Design review of the part shown in the three views and the two pictorial views. Dimensions are in mm from the part's minimum x, y and z. A direction names the side the tool comes from. Give positions to 0.01 mm unless a question says otherwise; leave off trailing zeros. Order: outer loops, then holes, each group sorted by start corner. A loop starts at its lowest first (then second) coordinate and runs counter-clockwise, first axis right, second up. Notation, with made-up numbers: (60, 76.25) -> (101, 76.25) arc R25 ccw to (101, 90.25) -> close; hole circle Ø10 at (69, 25). An arc over 180 degrees is marked (long way). Use one line per item in the form item = value.
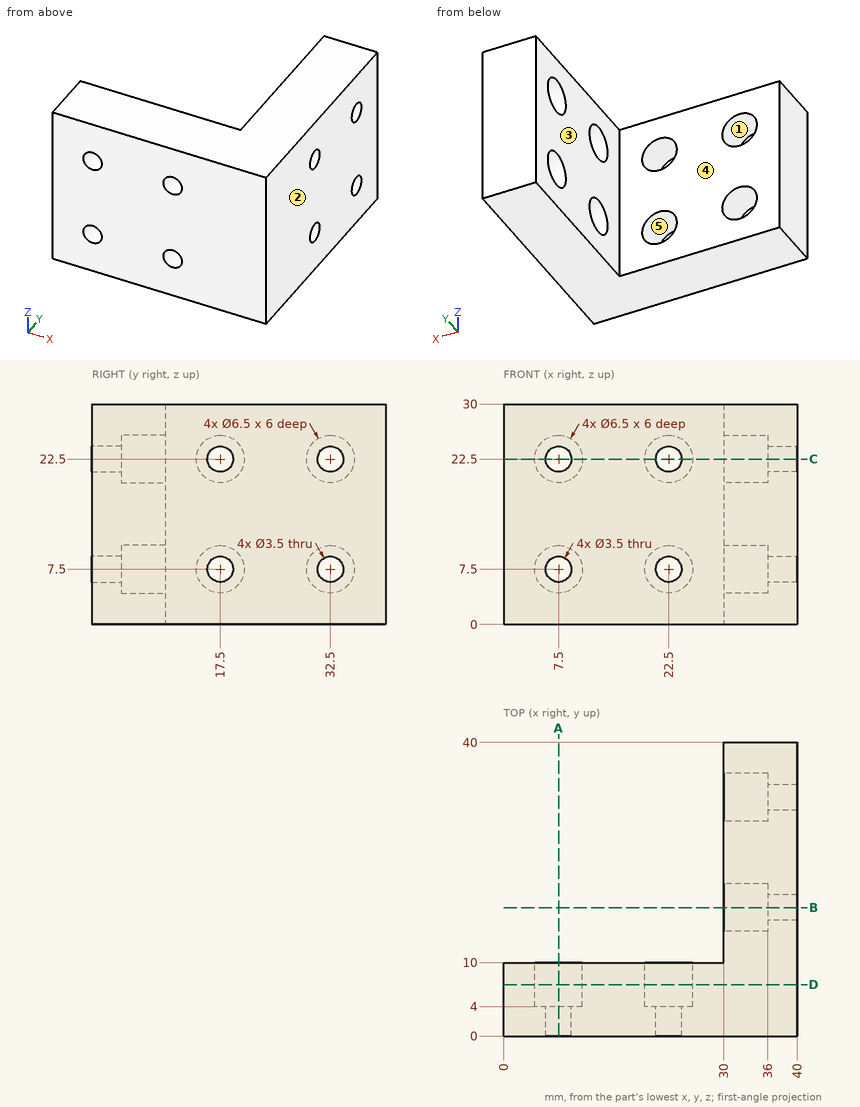
1. Add section C-C on z = 22.5. Count the separate pieces of the cut face and the enclosed holes in it, then the cut area to 3 significant figures.
Values:
separate_pieces = 5
enclosed_holes = 0
area = 488 mm^2
2. Tool access review of the marked faces 1 and 2: name each direction out of +Z, -Z, +X, -X, +Y, -Y from which nothing blocks a thin tool from reaching the whole face with its end or side.
Values:
face_1 = +Y
face_2 = +Z, -Z, +X, +Y, -Y
3. Add section D-D on y = 7. Give the boundary of the cut face in (x, z).
Values:
outline = (0, 0) -> (40, 0) -> (40, 30) -> (0, 30) -> close; hole circle Ø6.5 at (7.5, 7.5); hole circle Ø6.5 at (7.5, 22.5); hole circle Ø6.5 at (22.5, 7.5); hole circle Ø6.5 at (22.5, 22.5)
4. Add section A-A on x = 7.5. Give the boundary of the cut face in (y, z).
Values:
outline = (0, 0) -> (10, 0) -> (10, 4.25) -> (4, 4.25) -> (4, 5.75) -> (0, 5.75) -> close; (0, 9.25) -> (4, 9.25) -> (4, 10.75) -> (10, 10.75) -> (10, 19.25) -> (4, 19.25) -> (4, 20.75) -> (0, 20.75) -> close; (0, 24.25) -> (4, 24.25) -> (4, 25.75) -> (10, 25.75) -> (10, 30) -> (0, 30) -> close
5. For L1, parallel to Y at x = 37.35, z = 22.5; L2, parallel to X at y = 1, z = 22.5; L3, parallel to X at y = 6.05, z = 7.5, list the stretches that pass through material, from the lowest coordinate up.
Values:
L1 = 0 to 15.75, 19.25 to 30.75, 34.25 to 40
L2 = 0 to 5.75, 9.25 to 20.75, 24.25 to 40
L3 = 0 to 4.25, 10.75 to 19.25, 25.75 to 40
6. The part is to be moulded in two halves that separate along X. For the marked faces 3, 4 and 5, say which applies: +X half, -X half, draft (parallel to the pull), parting line (faces both ways), or undercut.
Values:
face_3 = -X half
face_4 = draft
face_5 = undercut
7. Add section B-B on y = 17.5. Give the boundary of the cut face in (x, z).
Values:
outline = (30, 0) -> (40, 0) -> (40, 5.75) -> (36, 5.75) -> (36, 4.25) -> (30, 4.25) -> close; (30, 10.75) -> (36, 10.75) -> (36, 9.25) -> (40, 9.25) -> (40, 20.75) -> (36, 20.75) -> (36, 19.25) -> (30, 19.25) -> close; (30, 25.75) -> (36, 25.75) -> (36, 24.25) -> (40, 24.25) -> (40, 30) -> (30, 30) -> close
8. For pin 1 Ø8.5 at (x, z) = (22.5, 7.5) entering from -Y; pin 2 Ø2 at (x, z) = (7.5, 21.5) entering from +Y; pin 3 Ø4 at (y, z) = (28, 26) entering from -X; pin 4 Ø10.5 at (x, z) = (22.5, 22.5) entering from +Y, all flat-tipped, find the tip position at first contact; note any pin that passes through.
Values:
pin_1 = 0
pin_2 = 4
pin_3 = 30
pin_4 = 10
